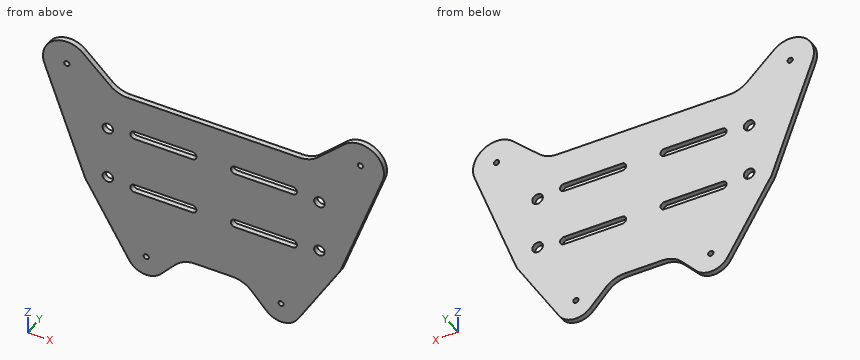
from build123d import *

# Parameters (mm, degrees)
SKETCH1_W           = 130
SKETCH1_H           = 90
BOSS_EXTRUDE2_DEPTH = 2
SKETCH2_R           = 2
CUT_EXTRUDE1_DEPTH  = 10
CUT_EXTRUDE3_DEPTH  = 10
SKETCH5_R           = 1
CUT_EXTRUDE4_DEPTH  = 10
CUT_EXTRUDE5_DEPTH  = 149.761308663
FILLET1_R           = 10


with BuildPart() as part:
    # Sketch1 → Boss-Extrude2 (new body)
    with BuildSketch(Plane(origin=(0, 0, 0), x_dir=(1, 0, 0), z_dir=(0, 1, 0))):
        with Locations((56.787418592, 40.403463793)):
            Rectangle(SKETCH1_W, SKETCH1_H)
    extrude(amount=BOSS_EXTRUDE2_DEPTH)

    # Sketch2 → Cut-Extrude1 (cut)
    with BuildSketch(Plane(origin=(0, 2, 0), x_dir=(1, 0, 0), z_dir=(0, 1, 0))):
        with Locations(Location((16.787418592, 50.403463793, 0), (0, 0, 270))):
            Circle(SKETCH2_R)
        with Locations(Location((16.787418592, 30.403463793, 0), (0, 0, 270))):
            Circle(SKETCH2_R)
        with Locations(Location((96.787418592, 50.403463793, 0), (0, 0, 270))):
            Circle(SKETCH2_R)
        with Locations(Location((96.787418592, 30.403463793, 0), (0, 0, 270))):
            Circle(SKETCH2_R)
    extrude(amount=-CUT_EXTRUDE1_DEPTH, mode=Mode.SUBTRACT)

    # Sketch4 → Cut-Extrude3 (cut)
    with BuildSketch(Plane(origin=(0, 2, 0), x_dir=(1, 0, 0), z_dir=(0, 1, 0))):
        with BuildLine():
            Line((26.787418592, 52.903463793), (48.787418592, 52.903463793))
            ThreePointArc((48.787418592, 52.903463793), (50.287418592, 51.403463793), (48.787418592, 49.903463793))
            Line((48.787418592, 49.903463793), (26.787418592, 49.903463793))
            ThreePointArc((26.787418592, 49.903463793), (25.287418592, 51.403463793), (26.787418592, 52.903463793))
        make_face()
        with BuildLine():
            Line((26.787418592, 30.903463793), (48.787418592, 30.903463793))
            ThreePointArc((48.787418592, 30.903463793), (50.287418592, 29.403463793), (48.787418592, 27.903463793))
            Line((48.787418592, 27.903463793), (26.787418592, 27.903463793))
            ThreePointArc((26.787418592, 27.903463793), (25.287418592, 29.403463793), (26.787418592, 30.903463793))
        make_face()
        with BuildLine():
            Line((64.787418592, 52.903463793), (86.787418592, 52.903463793))
            ThreePointArc((86.787418592, 52.903463793), (88.287418592, 51.403463793), (86.787418592, 49.903463793))
            Line((86.787418592, 49.903463793), (64.787418592, 49.903463793))
            ThreePointArc((64.787418592, 49.903463793), (63.287418592, 51.403463793), (64.787418592, 52.903463793))
        make_face()
        with BuildLine():
            Line((64.787418592, 30.903463793), (86.787418592, 30.903463793))
            ThreePointArc((86.787418592, 30.903463793), (88.287418592, 29.403463793), (86.787418592, 27.903463793))
            Line((86.787418592, 27.903463793), (64.787418592, 27.903463793))
            ThreePointArc((64.787418592, 27.903463793), (63.287418592, 29.403463793), (64.787418592, 30.903463793))
        make_face()
    extrude(amount=-CUT_EXTRUDE3_DEPTH, mode=Mode.SUBTRACT)

    # Sketch5 → Cut-Extrude4 (cut)
    with BuildSketch(Plane(origin=(0, 2, 0), x_dir=(1, 0, 0), z_dir=(0, 1, 0))):
        with Locations(Location((1.287418592, 9.403463793, 0), (0, 0, 270))):
            Circle(SKETCH5_R)
        with Locations(Location((112.287418592, 9.403463793, 0), (0, 0, 270))):
            Circle(SKETCH5_R)
        with Locations(Location((31.287418592, 77.903463793, 0), (0, 0, 270))):
            Circle(SKETCH5_R)
        with Locations(Location((82.287418592, 77.903463793, 0), (0, 0, 270))):
            Circle(SKETCH5_R)
    extrude(amount=-CUT_EXTRUDE4_DEPTH, mode=Mode.SUBTRACT)

    # Sketch6 → Cut-Extrude5 (cut, through all)
    with BuildSketch(Plane(origin=(0, 2, 0), x_dir=(1, 0, 0), z_dir=(0, 1, 0))):
        with BuildLine():
            Line((31.28741871, 85.403463793), (-8.212581408, 85.403463793))
            Line((-8.212581408, 85.403463793), (-8.212581408, -4.596536207))
            Line((-8.212581408, -4.596536207), (121.787418592, -4.596536207))
            Line((121.787418592, -4.596536207), (121.787418592, 85.403463793))
            Line((121.787418592, 85.403463793), (82.287418592, 85.403463793))
            ThreePointArc((82.287418592, 85.403463793), (86.000200188, 84.420000667), (88.739279438, 81.727531213))
            Line((88.739279438, 81.727531213), (104.673461226, 55.855633786))
            Line((104.673461226, 55.855633786), (120.652052787, 12.485170978))
            ThreePointArc((120.652052787, 12.485170978), (117.254615907, 2.001371169), (106.265325845, 2.830913046))
            Line((106.265325845, 2.830913046), (93.195977552, 14.805689748))
            Line((93.195977552, 14.805689748), (20.378859632, 14.805689748))
            Line((20.378859632, 14.805689748), (7.425097101, 2.787815466))
            ThreePointArc((7.425097103, 2.787815464), (-3.723088928, 1.897951505), (-7.176040156, 12.53519915))
            Line((-7.176040154, 12.53519915), (8.242814409, 54.204377623))
            Line((8.242814409, 54.204377623), (8.329286173, 54.347812353))
            ThreePointArc((8.329286173, 54.347812353), (8.794878375, 55.221885781), (9.350471922, 56.041700557))
            Line((9.350471922, 56.041700557), (24.835557745, 81.727531213))
            ThreePointArc((24.835557746, 81.727531212), (27.574637047, 84.420000696), (31.28741871, 85.403463793))
        make_face()
        with BuildLine():
            Line((82.287418592, 85.403463793), (31.28741871, 85.403463793))
            ThreePointArc((31.28741871, 85.403463793), (34.283566781, 84.779007119), (36.780790962, 83.00962282))
            Line((36.780790963, 83.009622821), (45.361476392, 73.77824166))
            Line((45.361476392, 73.77824166), (68.213360792, 73.77824166))
            Line((68.213360792, 73.77824166), (76.794046223, 83.009622821))
            ThreePointArc((76.794046223, 83.009622821), (79.291270457, 84.779007143), (82.287418592, 85.403463793))
        make_face()
    extrude(amount=-CUT_EXTRUDE5_DEPTH, mode=Mode.SUBTRACT)

    # Fillet1
    # the kernel refuses this fillet: 10 mm, written as the material it adds along each edge
    with BuildSketch(Plane(origin=(45.361476392, 2, -73.77824166), x_dir=(1, 0, 0), z_dir=(0, -1, 0))) as fillet1_piece_1:
        with BuildLine():
            CenterArc((FILLET1_R * 0.435768925154, -FILLET1_R), FILLET1_R, 90, 47.092151835)
            Line((-FILLET1_R * 0.296680724118, -FILLET1_R * 0.319178796393), (0, 0))
            Line((0, 0), (FILLET1_R * 0.435768925154, 0))
        make_face()
    extrude(amount=2)
    with BuildSketch(Plane(origin=(68.213360792, 2, -73.77824166), x_dir=(-1, 0, 0), z_dir=(0, -1, 0))) as fillet1_piece_2:
        with BuildLine():
            CenterArc((FILLET1_R * 0.435768925095, FILLET1_R), FILLET1_R, 222.907848171, 47.092151829)
            Line((-FILLET1_R * 0.296680724109, FILLET1_R * 0.31917879632), (0, 0))
            Line((0, 0), (FILLET1_R * 0.435768925095, 0))
        make_face()
    extrude(amount=2)
    with BuildSketch(Plane(origin=(93.195977552, 2, -14.805689748), x_dir=(0.7373075314629184, 0, 0.6755572544559473), z_dir=(0, -1, 0))) as fillet1_piece_3:
        with BuildLine():
            CenterArc((FILLET1_R * 0.388853005137, FILLET1_R), FILLET1_R, 227.502560825, 42.497439175)
            Line((-FILLET1_R * 0.286704249319, FILLET1_R * 0.262692468537), (0, 0))
            Line((0, 0), (FILLET1_R * 0.388853005137, 0))
        make_face()
    extrude(amount=2)
    with BuildSketch(Plane(origin=(20.378859632, 2, -14.805689748), x_dir=(1, 0, 0), z_dir=(0, -1, 0))) as fillet1_piece_4:
        with BuildLine():
            CenterArc((FILLET1_R * 0.392436109253, FILLET1_R), FILLET1_R, 227.146329541, 42.853670459)
            Line((-FILLET1_R * 0.287692200824, FILLET1_R * 0.2669069078), (0, 0))
            Line((0, 0), (FILLET1_R * 0.392436109253, 0))
        make_face()
    extrude(amount=2)
    # the kernel refuses this fillet: 10 mm, written as the material it takes off along each edge
    with BuildSketch(Plane(origin=(104.673461226, 4.496112329, -55.855633786), x_dir=(0.3457053588273583, 0, 0.9383431168171094), z_dir=(0, -1, 0))) as fillet1_2_piece_1:
        with BuildLine():
            CenterArc((FILLET1_R * 0.0998444931431, FILLET1_R), FILLET1_R, 258.596457336, 11.403542664)
            Line((-FILLET1_R * 0.0978734581483, FILLET1_R * 0.019741048632), (0, 0))
            Line((0, 0), (FILLET1_R * 0.0998444931431, 0))
        make_face()
    extrude(amount=6.992224657, mode=Mode.SUBTRACT)
    with BuildSketch(Plane(origin=(8.242814409, 3.565796653, -54.204377623), x_dir=(0.516298681525034, 0, -0.8564085890832199), z_dir=(0, -1, 0))) as fillet1_2_piece_2:
        with BuildLine():
            CenterArc((1.254824259, 9.940708785), FILLET1_R, 259.221695576, 4.53596152)
            Line((-0.615269231, 0.117127445), (0, 0))
            Line((0, 0), (0.167483992, 0))
        make_face()
    extrude(amount=5.131593306, mode=Mode.SUBTRACT)


solid = part.part
The model under review builds one solid part; all positions refer to its coordinate system, in mm. Give positions to 0.01 mm unless a question says otherwise; leave off trailing zeros. Order: outer loops, then holes, each group sorted by start corner. A loop starts at its lowest first (then second) coordinate and runs counter-clockwise, first axis right, second up. Notation, with made-up numbers: M 15,73 L 32,73 A7 cw 32,79 Z; hole C -4.5,52.5 d9. An arc over 180 degrees is marked long. Use one line per item in the form item = value. Start each with the question number.
Item 1: We need section B-B on x = 44. Give the boundary of the cut face in (y, z), plus the area to 3 significant figures.
Item 2: To check wall thickness, follow line 1 along Z through (x, y) = (73, 1.25); line 2 along Z through (x, y) = (98, 1.85); line 3 along X through (y, z) = (1.85, -51.5). State the ranges of each line that lie inside material, in increasing order. Write a range as from..to.
Item 3: Insertion check: pin 1 Ø10 at (x, z) = (59, -74.5) entering from -Y; pin 2 Ø0.6 at (x, y) = (33, 0.5) entering from -Z; pin 3 Ø1 at (x, y) = (52, 1) entering from +Z; pin 4 Ø1 at (x, y) = (59.5, 0.5) entering from -Z. Each pin has a flat end and moves straight along its axis. Give the tip position at first contact, or say it passes through.
Item 4: We need section A-A on z = -5.5. Give the boundary of the cut face in (x, y).
Item 5: We need section D-D on y = 1.25. Give the number of separate pieces and of enclosed holes in the cut face, plus the area to 3 significant figures.
Item 6: We need section C-C on z = -37. Give the boundary of the cut face in (x, y), plus the area to 3 significant figures.
Completed:
q1.outline = M 0,-75.58 L 2,-75.58 L 2,-52.9 L 0,-52.9 Z; M 0,-49.9 L 2,-49.9 L 2,-30.9 L 0,-30.9 Z; M 0,-27.9 L 2,-27.9 L 2,-14.81 L 0,-14.81 Z
q1.area = 110 mm²
q2.line_1 = -78.93..-52.9, -49.9..-30.9, -27.9..-14.81
q2.line_2 = -66.69..-51.99, -48.81..-31.99, -28.81..-10.4
q2.line_3 = 7.24..15.11, 18.46..25.29, 50.28..63.29, 88.28..95.11, 98.46..106.28
q3.pin_1 = 0
q3.pin_2 = -85.27
q3.pin_3 = -14.81
q3.pin_4 = -73.78
q4.outline = M -6.85,0 L 10.35,0 L 10.35,2 L -6.85,2 Z; M 103.35,0 L 120.3,0 L 120.3,2 L 103.35,2 Z
q5.separate_pieces = 1
q5.enclosed_holes = 12
q5.area = 6,640 mm²
q6.outline = M 1.88,0 L 111.62,0 L 111.62,2 L 1.88,2 Z
q6.area = 219 mm²
